Source: CAD feature listing. Evaluate the final solid. Frame: model axes, mm. A direction names the side the tool comes from. Give positions to 0.01 mm unless a question says otherwise; leave off trailing zeros. Loops run counter-clockwise (first coordinate to the right, second up) from the corner with the lowest first, then second, coordinate; pieces in that order, holes last. Notation, with made-up numbers: (25.25, -29) - (45.25, -29) arc R9 ccw to (45.25, -16) - close; hole circle Ø7 at (77.5, 18). An arc over 180 degrees is marked (long way). Write each question's results on one line, items separated by ' | '. Start each with the question number.
(1) Cut plane B-B on y = 22. Return the cut outline in (x, z).
(2) Cut plane A-A on x = -97.5. Give the number of separate pieces and of enclosed holes in the cut face, then the cut area to 3 significant figures.
(3) Material intervals for line 1 along X through (y, z) = (113.9, 37.5); line 2 along Z through (x, y) = (-97, 115); line 3 along X through (y, z) = (66.5, 0), sorted ascending. Write a range as [from, to].
(4) Contact query for flat-ended pins moving along their axis: pin 1 (1 mm diameter, centred on y = 70.5, z = 59, fed in from +X) (3 decimals); pin 2 (6.5 mm diameter, centred on x = 55, z = 55, fed in from -Y); pin 3 (0.5 mm diameter, centred on x = -105, y = 114.5, fed in from -Z). Output: stop coordinate, or through.
(5) Pull-direction query (Z, two-part tool) for faces 1 (the cylindrical face through (-101.049, 31.521, -35.654)), 2 (the cylindrical face through (-71.797, 101.4, -71.486)), 3 (the flat face through (77.5, 99, 1)); classes: pulls with the +Z half, pulls with the -Z half, needs draft (parallel to the pull), parting line crosses it, or undercut.
(6) Reachability of faces 4 (the flat face through (-97, 116, -1)), 5 (the flat face through (-43.24, 198, -30)), 6 (the flat face through (-77.5, 15, 1)), 7 (the cylindrical face through (-53.154, 12.675, -51.451)) from +Z, -Z, +X, -X, +Y, -Y: full face, straight path, thin tool, end or side. Return the list, or none.
(7) Cut plane C-C on y = 159. Return the cut outline in (x, z), then the cut area to 3 significant figures.
from build123d import *

# Parameters (mm, degrees)
SZKIC1_W                       = 155
SZKIC1_H                       = 155
DODANIE_WYCI_GNI_CIE1_DEPTH    = 200
SZKIC2_W                       = 19
SZKIC2_H                       = 15
SZKIC2_W_2                     = 15
WYTNIJ_WYCI_GNI_CIE1_DEPTH     = 90
ZAOKR_GLENIE1_R                = 20
SZKIC4_R                       = 8
DODANIE_WYCI_GNI_CIE2_DEPTH    = 10
ZAOKR_GLENIE2_R                = 2
SZKIC5_W                       = 135
SZKIC5_H                       = 170
WYTNIJ_WYCI_GNI_CIE2_DEPTH     = 120
SZKIC6_R                       = 10
DODANIE_WYCI_GNI_CIE3_DEPTH    = 80
SZKIC8_W                       = 115
SZKIC8_H                       = 3
DODANIE_WYCI_GNI_CIE4_DEPTH    = 40
SZKIC9_R                       = 4
WYTNIJ_WYCI_GNI_CIE3_DEPTH     = 100
ZAOKR_GLENIE3_R                = 1
OTWORY_USTALAJ_CE_8_0MM1_D     = 8
OTWORY_USTALAJ_CE_8_0MM1_DEPTH = 25
ZAOKR_GLENIE4_R                = 10
ZAOKR_GLENIE5_R                = 5


with BuildPart() as part:
    # Szkic1 → Dodanie-wyciągnięcie1 (new body)
    with BuildSketch(Plane(origin=(0, 0, 0), x_dir=(1, 0, 0), z_dir=(0, 1, 0))):
        Rectangle(SZKIC1_W, SZKIC1_H)
    extrude(amount=DODANIE_WYCI_GNI_CIE1_DEPTH)

    # Szkic2 → Wytnij-wyciągnięcie1 (cut)
    with BuildSketch(Plane(origin=(0, 200, 0), x_dir=(1, 0, 0), z_dir=(0, 1, 0))):
        with BuildLine():
            Line((-58.240160679, 43), (-58.240160679, -43))
            ThreePointArc((-58.240160679, -43), (-50.740160679, -50.5), (-43.240160679, -43))
            Line((-43.240160679, -43), (-43.240160679, -7.5))
            Line((-43.240160679, -7.5), (-43.240160679, 7.5))
            Line((-43.240160679, 7.5), (-43.240160679, 43))
            ThreePointArc((-43.240160679, 43), (-50.740160679, 50.5), (-58.240160679, 43))
        make_face()
        with Locations((-33.740160679, 0)):
            Rectangle(SZKIC2_W, SZKIC2_H)
        with BuildLine():
            Line((-9.240160679, -7.5), (-24.240160679, -7.5))
            Line((-24.240160679, -7.5), (-24.240160679, -43))
            ThreePointArc((-24.240160679, -43), (-16.740160679, -50.5), (-9.240160679, -43))
            Line((-9.240160679, -43), (-9.240160679, -7.5))
        make_face()
        with Locations((-16.740160679, 0)):
            Rectangle(SZKIC2_W_2, SZKIC2_H)
        with BuildLine():
            Line((-24.240160679, 43), (-24.240160679, 7.5))
            Line((-24.240160679, 7.5), (-9.240160679, 7.5))
            Line((-9.240160679, 7.5), (-9.240160679, 43))
            ThreePointArc((-9.240160679, 43), (-16.740160679, 50.5), (-24.240160679, 43))
        make_face()
        Polygon((-9.240160679, 7.5), (-9.240160679, -7.5), (9.759839321, -7.5), (9.759839321, -4.6e-08), (9.759839321, 7.5), align=None)
        with BuildLine():
            Line((17.259839321, -7.5), (9.759839321, -7.5))
            Line((9.759839321, -7.5), (9.759839321, -43))
            ThreePointArc((9.759839321, -43), (17.259839321, -50.5), (24.759839321, -43))
            Line((24.759839321, -43), (24.759839321, -8.554286585))
            ThreePointArc((24.759839321, -8.554286585), (21.046708747, -7.764861006), (17.259839321, -7.5))
        make_face()
        with BuildLine():
            Line((9.759839321, -4.6e-08), (9.759839321, -7.5))
            Line((9.759839321, -7.5), (17.259839321, -7.5))
            ThreePointArc((17.259839321, -7.5), (11.956538478, -5.303300875), (9.759839321, -4.6e-08))
        make_face()
        with BuildLine():
            Line((17.259839321, 7.5), (9.759839321, 7.5))
            Line((9.759839321, 7.5), (9.759839321, -4.6e-08))
            ThreePointArc((9.759839321, -4.6e-08), (11.956538445, 5.303300843), (17.259839321, 7.5))
        make_face()
        with BuildLine():
            Line((9.759839321, 43), (9.759839321, 7.5))
            Line((9.759839321, 7.5), (17.259839321, 7.5))
            ThreePointArc((17.259839321, 7.5), (21.024851006, 7.331726309), (24.759839321, 6.828247104))
            Line((24.759839321, 6.828247104), (24.759839321, 43))
            ThreePointArc((24.759839321, 43), (17.259839321, 50.5), (9.759839321, 43))
        make_face()
        with BuildLine():
            ThreePointArc((17.259839321, 7.5), (11.956538445, 5.303300843), (9.759839321, -4.6e-08))
            ThreePointArc((9.759839321, -4.6e-08), (11.956538478, -5.303300875), (17.259839321, -7.5))
            Line((17.259839321, -7.5), (17.259839321, 7.5))
        make_face()
        with BuildLine():
            Line((17.259839321, 7.5), (17.259839321, -7.5))
            ThreePointArc((17.259839321, -7.5), (21.046708747, -7.764861006), (24.759839321, -8.554286585))
            Line((24.759839321, -8.554286585), (24.759839321, 6.828247104))
            ThreePointArc((24.759839321, 6.828247104), (21.024851006, 7.331726309), (17.259839321, 7.5))
        make_face()
        with BuildLine():
            Line((24.759839321, 6.828247104), (24.759839321, -8.554286585))
            ThreePointArc((24.759839321, -8.554286585), (40.799428369, -21.067870737), (43.675059249, -41.207109854))
            ThreePointArc((43.675059249, -41.207109854), (49.164719818, -50.282550715), (58.240160679, -44.792890146))
            ThreePointArc((58.240160679, -44.792890146), (52.668465989, -11.738702912), (24.759839321, 6.828247104))
        make_face()
    extrude(amount=-WYTNIJ_WYCI_GNI_CIE1_DEPTH, mode=Mode.SUBTRACT)

    # Zaokrąglenie1
    zaokr_glenie1_edges = [part.edges().sort_by_distance(p)[0] for p in [
        (77.5, 100, 77.5),
        (-77.5, 100, 77.5),
        (-77.5, 100, -77.5),
        (77.5, 100, -77.5),
    ]]
    fillet(zaokr_glenie1_edges, radius=ZAOKR_GLENIE1_R)

    # Szkic4 → Dodanie-wyciągnięcie2 (add)
    with BuildSketch(Plane(origin=(0, 200, 0), x_dir=(1, 0, 0), z_dir=(0, 1, 0))):
        with Locations(Location((-64.571067812, -64.571067812, 0), (0, 0, 90))):
            Circle(SZKIC4_R)
        with Locations(Location((-64.571067812, 64.571067812, 0), (0, 0, 90))):
            Circle(SZKIC4_R)
        with Locations(Location((64.571067812, 64.571067812, 0), (0, 0, 90))):
            Circle(SZKIC4_R)
        with Locations(Location((64.571067812, -64.571067812, 0), (0, 0, 90))):
            Circle(SZKIC4_R)
    extrude(amount=DODANIE_WYCI_GNI_CIE2_DEPTH)

    # Zaokrąglenie2
    zaokr_glenie2_edges = [part.edges().sort_by_distance(p)[0] for p in [
        (-64.571067812, 210, 72.571067812),
        (-64.571067812, 210, -56.571067812),
        (64.571067812, 210, -56.571067812),
        (64.571067812, 210, 72.571067812),
    ]]
    fillet(zaokr_glenie2_edges, radius=ZAOKR_GLENIE2_R)

    # Szkic5 → Wytnij-wyciągnięcie2 (cut)
    with BuildSketch(Plane.XY.offset(57.5)):
        with Locations((0, 110)):
            Rectangle(SZKIC5_W, SZKIC5_H)
    extrude(amount=-WYTNIJ_WYCI_GNI_CIE2_DEPTH, mode=Mode.SUBTRACT)

    # Szkic6 → Dodanie-wyciągnięcie3 (add)
    with BuildSketch(Plane(origin=(0, 25, 0), x_dir=(1, 0, 0), z_dir=(0, 1, 0))):
        with Locations(Location((-16.740160679, 0, 0), (0, 0, 90))):
            Circle(SZKIC6_R)
    extrude(amount=DODANIE_WYCI_GNI_CIE3_DEPTH)

    # Szkic7 → Wycięcie-obrót1 (revolve, cut)
    with BuildSketch(Plane(origin=(0, 105, 0), x_dir=(1, 0, 0), z_dir=(0, 1, 0))):
        with BuildLine():
            Line((-16.740160679, 8), (-16.740160679, -8))
            ThreePointArc((-16.740160679, -8), (-8.740160679, 0), (-16.740160679, 8))
        make_face()
    revolve(axis=Axis((-16.740160679, 105, -8), (0, 0, 1)), mode=Mode.SUBTRACT)

    # Szkic8 → Dodanie-wyciągnięcie4 (add)
    with BuildSketch(Plane.ZY.offset(77.5)):
        with Locations((0, 114.5)):
            Rectangle(SZKIC8_W, SZKIC8_H)
        with Locations((0, 31.5)):
            Rectangle(SZKIC8_W, SZKIC8_H)
    extrude(amount=DODANIE_WYCI_GNI_CIE4_DEPTH)

    # Szkic9 → Wytnij-wyciągnięcie3 (cut)
    with BuildSketch(Plane(origin=(0, 116, 0), x_dir=(1, 0, 0), z_dir=(0, 1, 0))):
        with Locations(Location((-97.5, 37.5, 0), (0, 0, 270))):
            Circle(SZKIC9_R)
        with Locations(Location((-97.5, -37.5, 0), (0, 0, 270))):
            Circle(SZKIC9_R)
    extrude(amount=-WYTNIJ_WYCI_GNI_CIE3_DEPTH, mode=Mode.SUBTRACT)

    # Zaokrąglenie3
    zaokr_glenie3_edges = [part.edges().sort_by_distance(p)[0] for p in [
        (-97.5, 116, -57.5),
        (-97.5, 113, -57.5),
        (-97.5, 113, 57.5),
        (-97.5, 116, 57.5),
        (-117.5, 113, 0),
        (-117.5, 116, 0),
        (-97.5, 30, 57.5),
        (-97.5, 33, 57.5),
        (-97.5, 33, -57.5),
        (-97.5, 30, -57.5),
        (-117.5, 33, 0),
        (-117.5, 30, 0),
    ]]
    fillet(zaokr_glenie3_edges, radius=ZAOKR_GLENIE3_R)

    # Otwory ustalające Ø8.0mm1
    with Locations(Plane(origin=(0, 0, 0), x_dir=(-1, 0, 0), z_dir=(0, -1, 0))):
        with Locations((55, 55), (55, -55), (-55, -55), (-55, 55)):
            Hole(OTWORY_USTALAJ_CE_8_0MM1_D / 2, depth=OTWORY_USTALAJ_CE_8_0MM1_DEPTH)

    # Zaokrąglenie4
    # the kernel refuses this fillet: 10 mm, written as the material it takes off along each edge
    with BuildSketch(Plane(origin=(-9.240160679, 225, 7.5), x_dir=(0, 0, 1), z_dir=(0, -1, 0)), Plane(origin=(9.759839321, 225, 7.5), x_dir=(-1, 0, 0), z_dir=(0, -1, 0)), Plane(origin=(-24.240160679, 225, 7.5), x_dir=(-1, 0, 0), z_dir=(0, -1, 0)), Plane(origin=(-43.240160679, 225, 7.5), x_dir=(0, 0, 1), z_dir=(0, -1, 0))) as zaokr_glenie4_piece_1:
        with BuildLine():
            CenterArc((ZAOKR_GLENIE4_R, -ZAOKR_GLENIE4_R), ZAOKR_GLENIE4_R, 90, 90)
            Line((0, -ZAOKR_GLENIE4_R), (0, 0))
            Line((0, 0), (ZAOKR_GLENIE4_R, 0))
        make_face()
    extrude(amount=55, mode=Mode.SUBTRACT)
    with BuildSketch(Plane(origin=(9.759839321, 225, -7.5), x_dir=(-1, 0, 0), z_dir=(0, -1, 0)), Plane(origin=(-9.240160679, 225, -7.5), x_dir=(0, 0, -1), z_dir=(0, -1, 0)), Plane(origin=(-24.240160679, 225, -7.5), x_dir=(-1, 0, 0), z_dir=(0, -1, 0)), Plane(origin=(-43.240160679, 225, -7.5), x_dir=(0, 0, -1), z_dir=(0, -1, 0))) as zaokr_glenie4_piece_2:
        with BuildLine():
            CenterArc((ZAOKR_GLENIE4_R, ZAOKR_GLENIE4_R), ZAOKR_GLENIE4_R, 180, 90)
            Line((0, ZAOKR_GLENIE4_R), (0, 0))
            Line((0, 0), (ZAOKR_GLENIE4_R, 0))
        make_face()
    extrude(amount=55, mode=Mode.SUBTRACT)

    # Zaokrąglenie5
    zaokr_glenie5_edges = [part.edges().sort_by_distance(p)[0] for p in [
        (24.759839321, 197.5, 8.554286585),
        (24.759839321, 197.5, -6.828247104),
    ]]
    fillet(zaokr_glenie5_edges, radius=ZAOKR_GLENIE5_R)


solid = part.part
Ans:
1) outline: (-77.5, -57.5) arc R20 ccw to (-57.5, -77.5) - (57.5, -77.5) arc R20 ccw to (77.5, -57.5) - (77.5, 57.5) arc R20 ccw to (57.5, 77.5) - (-57.5, 77.5) arc R20 ccw to (-77.5, 57.5) - close; hole circle Ø8 at (-55, -55); hole circle Ø8 at (-55, 55); hole circle Ø8 at (55, -55); hole circle Ø8 at (55, 55)
2) separate pieces: 6 | enclosed holes: 0 | area: 592 mm^2
3) line 1: [-117.49, -101.5], [-93.5, -67.5], [67.5, 77.5] | line 2: [-57.5, -41.47], [-33.53, 33.53], [41.47, 57.5] | line 3: [-77.5, -67.5], [-26.74, -6.74], [67.5, 77.5]
4) pin 1: x = 77.475 | pin 2: y = 25 | pin 3: z = -57.5
5) face 1: undercut | face 2: pulls with the -Z half | face 3: needs draft
6) face 4: +Z, -Z, -X, +Y | face 5: +Y | face 6: +Z, -Z, -X, -Y | face 7: -Y
7) outline: (-77.5, -57.5) arc R20 ccw to (-57.5, -77.5) - (57.5, -77.5) arc R20 ccw to (77.5, -57.5) - (77.5, 57.5) arc R20 ccw to (57.5, 77.5) - (-57.5, 77.5) arc R20 ccw to (-77.5, 57.5) - close; hole (-67.5, -62.5) - (67.5, -62.5) - (67.5, 57.5) - (-67.5, 57.5) - close | area: 7,480 mm^2
